```python
from build123d import *

# Parameters (mm, degrees)
SKETCH1_W           = 7.5
SKETCH1_H           = 8
SKETCH1_H_2         = 10
SKETCH1_W_2         = 30
BOSS_EXTRUDE1_DEPTH = 2
SKETCH2_W           = 45
SKETCH2_H           = 30
BOSS_EXTRUDE2_DEPTH = 2


with BuildPart() as part:
    # Sketch1 → Boss-Extrude1 (new body)
    with BuildSketch(Plane.XY):
        with Locations((-18.75, 90)):
            Rectangle(SKETCH1_W, SKETCH1_H)
        with Locations((-18.75, 81)):
            Rectangle(SKETCH1_W, SKETCH1_H_2)
        with Locations((-18.75, 72)):
            Rectangle(SKETCH1_W, SKETCH1_H)
        with Locations((-18.75, 63)):
            Rectangle(SKETCH1_W, SKETCH1_H_2)
        with Locations((-18.75, 54)):
            Rectangle(SKETCH1_W, SKETCH1_H)
        with Locations((-18.75, 45)):
            Rectangle(SKETCH1_W, SKETCH1_H_2)
        with Locations((0, 90)):
            Rectangle(SKETCH1_W_2, SKETCH1_H)
        with Locations((18.75, 90)):
            Rectangle(SKETCH1_W, SKETCH1_H)
        with Locations((18.75, 81)):
            Rectangle(SKETCH1_W, SKETCH1_H_2)
        with Locations((18.75, 72)):
            Rectangle(SKETCH1_W, SKETCH1_H)
        with Locations((0, 72)):
            Rectangle(SKETCH1_W_2, SKETCH1_H)
        with Locations((0, 54)):
            Rectangle(SKETCH1_W_2, SKETCH1_H)
        with Locations((18.75, 54)):
            Rectangle(SKETCH1_W, SKETCH1_H)
        with Locations((18.75, 63)):
            Rectangle(SKETCH1_W, SKETCH1_H_2)
        with Locations((18.75, 45)):
            Rectangle(SKETCH1_W, SKETCH1_H_2)
        with Locations((18.75, 36)):
            Rectangle(SKETCH1_W, SKETCH1_H)
        with Locations((0, 36)):
            Rectangle(SKETCH1_W_2, SKETCH1_H)
        with Locations((-18.75, 36)):
            Rectangle(SKETCH1_W, SKETCH1_H)
        with Locations((-18.75, 27)):
            Rectangle(SKETCH1_W, SKETCH1_H_2)
        with Locations((-18.75, 18)):
            Rectangle(SKETCH1_W, SKETCH1_H)
        with Locations((-18.75, 9)):
            Rectangle(SKETCH1_W, SKETCH1_H_2)
        with Locations((-18.75, 0)):
            Rectangle(SKETCH1_W, SKETCH1_H)
        Rectangle(SKETCH1_W_2, SKETCH1_H)
        with Locations((18.75, 0)):
            Rectangle(SKETCH1_W, SKETCH1_H)
        with Locations((18.75, 9)):
            Rectangle(SKETCH1_W, SKETCH1_H_2)
        with Locations((18.75, 18)):
            Rectangle(SKETCH1_W, SKETCH1_H)
        with Locations((0, 18)):
            Rectangle(SKETCH1_W_2, SKETCH1_H)
        with Locations((18.75, 27)):
            Rectangle(SKETCH1_W, SKETCH1_H_2)
        with Locations((-18.75, -9)):
            Rectangle(SKETCH1_W, SKETCH1_H_2)
        with Locations((-18.75, -18)):
            Rectangle(SKETCH1_W, SKETCH1_H)
        with Locations((-18.75, -27)):
            Rectangle(SKETCH1_W, SKETCH1_H_2)
        with Locations((-18.75, -36)):
            Rectangle(SKETCH1_W, SKETCH1_H)
        with Locations((-18.75, -45)):
            Rectangle(SKETCH1_W, SKETCH1_H_2)
        with Locations((0, -36)):
            Rectangle(SKETCH1_W_2, SKETCH1_H)
        with Locations((0, -18)):
            Rectangle(SKETCH1_W_2, SKETCH1_H)
        with Locations((18.75, -18)):
            Rectangle(SKETCH1_W, SKETCH1_H)
        with Locations((18.75, -9)):
            Rectangle(SKETCH1_W, SKETCH1_H_2)
        with Locations((18.75, -27)):
            Rectangle(SKETCH1_W, SKETCH1_H_2)
        with Locations((18.75, -36)):
            Rectangle(SKETCH1_W, SKETCH1_H)
        with Locations((-18.75, -54)):
            Rectangle(SKETCH1_W, SKETCH1_H)
        with Locations((-18.75, -63)):
            Rectangle(SKETCH1_W, SKETCH1_H_2)
        with Locations((-18.75, -72)):
            Rectangle(SKETCH1_W, SKETCH1_H)
        with Locations((-18.75, -81)):
            Rectangle(SKETCH1_W, SKETCH1_H_2)
        with Locations((-18.75, -90)):
            Rectangle(SKETCH1_W, SKETCH1_H)
        with Locations((0, -90)):
            Rectangle(SKETCH1_W_2, SKETCH1_H)
        with Locations((18.75, -90)):
            Rectangle(SKETCH1_W, SKETCH1_H)
        with Locations((18.75, -81)):
            Rectangle(SKETCH1_W, SKETCH1_H_2)
        with Locations((18.75, -72)):
            Rectangle(SKETCH1_W, SKETCH1_H)
        with Locations((18.75, -63)):
            Rectangle(SKETCH1_W, SKETCH1_H_2)
        with Locations((18.75, -54)):
            Rectangle(SKETCH1_W, SKETCH1_H)
        with Locations((18.75, -45)):
            Rectangle(SKETCH1_W, SKETCH1_H_2)
        with Locations((0, -54)):
            Rectangle(SKETCH1_W_2, SKETCH1_H)
        with Locations((0, -72)):
            Rectangle(SKETCH1_W_2, SKETCH1_H)
    extrude(amount=BOSS_EXTRUDE1_DEPTH)

    # Sketch2 → Boss-Extrude2 (add)
    with BuildSketch(Plane.XY.offset(2)):
        with Locations((0, -109)):
            Rectangle(SKETCH2_W, SKETCH2_H)
    extrude(amount=-BOSS_EXTRUDE2_DEPTH)


solid = part.part
```
CAD build for the part. Positions are in the model's coordinates, mm. Round coordinates to 2 decimals unless told otherwise and drop trailing zeros. Order: outer loops, then holes, each group sorted by start corner. A loop starts at its lowest first (then second) coordinate and runs counter-clockwise, first axis right, second up. Notation, with made-up numbers: (-19.75, -6) -> (6.25, -6) arc R8 cw to (6.25, 2) -> close; hole circle Ø10 at (66, -27). An arc over 180 degrees is marked (long way). Write item = value, one per line.
(1) Drill centre line: L1, parallel to X at y = 6, z = 0.55. Where is it in solid material? Low to high.
Answers follow:
L1 = -22.5 to -15, 15 to 22.5
(2) Cut at B-B (x = -3.5). State how many separate pieces and enclosed holes the cut face has, plus the area to 3 significant figures.
Answers follow:
separate_pieces = 11
enclosed_holes = 0
area = 236 mm²
(3) Cut at A-A (y = 47). Write the cut outline in (x, z), plus the area to 3 significant figures.
Answers follow:
outline = (-22.5, 0) -> (-15, 0) -> (-15, 2) -> (-22.5, 2) -> close; (15, 0) -> (22.5, 0) -> (22.5, 2) -> (15, 2) -> close
area = 30.0 mm²
